Geometry: final body of the model. Coordinates: model frame, mm. A direction names the side the tool comes from. Round coordinates to 2 decimals unless told otherwise and drop trailing zeros. Loops run counter-clockwise (first coordinate to the right, second up) from the corner with the lowest first, then second, coordinate; pieces in that order, holes last. Notation, with made-up numbers: M -33.5,-0.5 L -10.5,-0.5 A21 ccw -10.5,22.5 Z; hole C 25,-0.5 d4. An arc over 180 degrees is marked long. Answer as a JSON object with one key per item and string values.
```python
from build123d import *

# Parameters (mm, degrees)
F0_R     = 2.25
F0_R_2   = 6
F1_DEPTH = 10
F2_R     = 12
F2_R_2   = 6
F3_DEPTH = 30
F4_R     = 2
F5_R     = 0.5


with BuildPart() as f1:
    # F0 (on Top) → F1 (new body)
    with BuildSketch(Plane.XY):
        with BuildLine():
            Line((-13.228757, -15), (13.228757, -15))
            ThreePointArc((13.228757, -15), (20, 0), (13.228757, 15))
            Line((13.228757, 15), (-13.228757, 15))
            ThreePointArc((-13.228757, 15), (-20, 0), (-13.228757, -15))
        make_face()
        with Locations((-11.313708, -11.313708)):
            Circle(F0_R, mode=Mode.SUBTRACT)
        with Locations((-16, 0)):
            Circle(F0_R, mode=Mode.SUBTRACT)
        Circle(F0_R_2, mode=Mode.SUBTRACT)
        with Locations((11.313708, -11.313708)):
            Circle(F0_R, mode=Mode.SUBTRACT)
        with Locations((16, 0)):
            Circle(F0_R, mode=Mode.SUBTRACT)
        with Locations((-11.313708, 11.313708)):
            Circle(F0_R, mode=Mode.SUBTRACT)
        with Locations((11.313708, 11.313708)):
            Circle(F0_R, mode=Mode.SUBTRACT)
    extrude(amount=F1_DEPTH)

    # F2 (on face) → F3 (join)
    with BuildSketch(Plane.XY.offset(10)):
        Circle(F2_R)
        Circle(F2_R_2, mode=Mode.SUBTRACT)
    extrude(amount=F3_DEPTH)

    # F4
    f4_edges = [f1.edges().sort_by_distance(p)[0] for p in [
        (-13.228757, -15, 5),
        (13.228757, -15, 5),
        (13.228757, 15, 5),
        (-13.228757, 15, 5),
    ]]
    fillet(f4_edges, radius=F4_R)

    # F5
    f5_edges = [f1.edges().sort_by_distance(p)[0] for p in [
        (-12, 0, 40),
        (20, 0, 10),
        (20, 0, 0),
        (-6, 0, 40),
        (-6, 0, 0),
    ]]
    fillet(f5_edges, radius=F5_R)


solid = f1.part
```
1) Cut plane C-C on z = 3. Return the cut outline in (x, y), and give its area (3 significant figures).
Geometry results:
{"outline": "M -13.83,-14.44 A2 ccw -12.45,-15 L 12.45,-15 A2 ccw 13.83,-14.44 A20 ccw 13.83,14.44 A2 ccw 12.45,15 L -12.45,15 A2 ccw -13.83,14.44 A20 ccw Z; hole C -16,0 d4.5; hole C -11.31,-11.31 d4.5; hole C -11.31,11.31 d4.5; hole C 0,0 d12; hole C 11.31,-11.31 d4.5; hole C 11.31,11.31 d4.5; hole C 16,0 d4.5", "area": "866 mm2"}
2) First-contact query: pin 1 (10 mm diameter, centred on y = 5.5, z = 26.5, fed in from -X); pin 2 (5 mm diameter, centred on x = 16, y = 0, fed in from +Z); pin 3 (12 mm diameter, centred on y = -10, z = 28, fed in from -X); pin 4 (11 mm diameter, centred on x = 0, y = 0, fed in from +Z). Flat tips, straight axial feed; report the tip coordinate or a pass-through.
Geometry results:
{"pin 1": "x = -11.99", "pin 2": "z = 10", "pin 3": "x = -11.31", "pin 4": "through"}
3) Cut plane D-D on z = 25. Return the cut outline in (x, y), and give its area (3 significant figures).
Geometry results:
{"outline": "C 0,0 d24; hole C 0,0 d12", "area": "339 mm2"}
4) Cut plane A-A on y = 0. Count the separate pieces of the cut face and the enclosed holes in it, and give its area (3 significant figures).
Geometry results:
{"separate pieces": "4", "enclosed holes": "0", "area": "549 mm2"}
5) Line query: probe 1 along X at (y, z) = (-1.75, 4.5); probe 2 along Y at (x, z) = (-10.5, 5.5); probe 3 along Z at (x, y) = (17, -9). Output: solid intervals per line, ascending.
Geometry results:
{"probe 1": "-19.92 to -17.41, -14.59 to -5.74, 5.74 to 14.59, 17.41 to 19.92", "probe 2": "-15 to -13.41, -9.22 to 9.22, 13.41 to 15", "probe 3": "0 to 10"}
6) Set-up query: faces 1 (the face through (-13, 0, 10)), 2 (the face through (13.21, -14.85, 5.06)). Return all of +Z, -Z, +X, -X, +Y, -Y with unobstructed straight access to the full face (end or side cutting, diameter ignored); none if empty.
Geometry results:
{"face 1": "+Z", "face 2": "+Z, -Z, +X, -Y"}
7) Pull-direction query (X, two-part tool) for faces 3 (the face through (-13.21, -14.85, 5.06)), 4 (the face through (13.19, 14.86, 5.06)), 5 (the face through (11.021, -9.083, 4.93)); classes: +X half, -X half, draft (parallel to the pull), parting line (faces both ways), or undercut.
Geometry results:
{"face 3": "-X half", "face 4": "+X half", "face 5": "undercut"}
8) Cut plane B-B on x = 0. Return the cut outline in (y, z), and give its area (3 significant figures).
Geometry results:
{"outline": "M -15,0.5 A0.5 ccw -14.5,0 L -6.5,0 A0.5 ccw -6,0.5 L -6,39.5 A0.5 ccw -6.5,40 L -11.5,40 A0.5 ccw -12,39.5 L -12,10 L -14.5,10 A0.5 ccw -15,9.5 Z; M 6,0.5 A0.5 ccw 6.5,0 L 14.5,0 A0.5 ccw 15,0.5 L 15,9.5 A0.5 ccw 14.5,10 L 12,10 L 12,39.5 A0.5 ccw 11.5,40 L 6.5,40 A0.5 ccw 6,39.5 Z", "area": "539 mm2"}
